Source: CAD feature listing. Evaluate the final solid. Frame: model axes, mm. Face numbers are marked on the shaded views. A direction names the side the tool comes from. Round coordinates to 2 decimals unless told otherwise and drop trailing zeros. Order: outer loops, then holes, each group sorted by start corner. A loop starts at its lowest first (then second) coordinate and runs counter-clockwise, first axis right, second up. Notation, with made-up numbers: M 27.5,63 L 44.5,63 A13 cw 44.5,70 Z; hole C 73.25,-23 d11. An arc over 180 degrees is marked long. Answer in a Markdown table with one row per item. Add a question column.
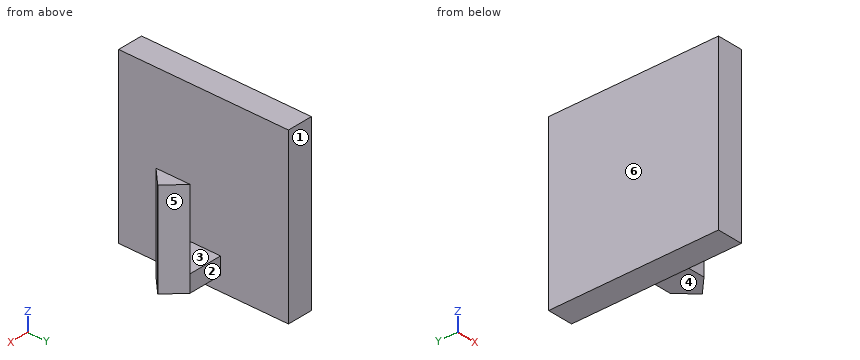
Autodesk Inventor part; units mm, degrees
ref_plane "YZ Plane" through (0, 0, 0) normal (1, 0, 0) x (0, 1, 0)
ref_plane "XZ Plane" through (0, 0, 0) normal (0, 1, 0) x (-1, 0, 0)
ref_plane "XY Plane" through (0, 0, 0) normal (0, 0, 1) x (1, 0, 0)
sketch "Esquisse1" plane through (0, 0, 0) normal (1, 0, 0) x (0, 1, 0)
  line L0 (5.4849, 2.6087) -> (-4.5151, 2.6087)
  line L1 (-4.5151, 2.6087) -> (-4.5151, -7.3913)
  line L2 (-4.5151, -7.3913) -> (5.4849, -7.3913)
  line L3 (5.4849, -7.3913) -> (5.4849, 2.6087)
  point P0 (0, 0)
  dimension "d0" = 10
  dimension "d1" = 10
extrude "Extrusion1" add sketch "Esquisse1" along normal blind 1.5
sketch "Esquisse2" plane through (1.5, 0, 0) normal (1, 0, 0) x (0, 0, -1)
  line L0 (5.5438, 1.4849) -> (6.5438, 1.4849)
  line L1 (6.5438, 1.4849) -> (6.5438, -0.5151)
  line L2 (6.5438, -0.5151) -> (5.5438, -0.5151)
  line L3 (5.5438, -0.5151) -> (5.5438, 1.4849)
  line L4 (7.3913, 5.4849) -> (-2.6087, 5.4849)
  point P0 (0, 0)
  dimension "d4" = 1
  dimension "d5" = 2
  dimension "d6" = 4
extrude "Extrusion2" add sketch "Esquisse2" along normal blind 2
sketch "Esquisse3" plane through (3.5, 0, 0) normal (1, 0, 0) x (0, 0, -1)
  line L0 (6.5438, 1.4849) -> (6.5438, -0.5151)
  line L1 (6.5438, 1.4849) -> (0.9284, 1.4849)
  line L2 (0.9284, 1.4849) -> (0.9284, -0.5151)
  line L3 (0.9284, -0.5151) -> (6.5438, -0.5151)
  line L4 (6.5438, -0.5151) -> (6.5438, 1.4849)
  point P0 (0, 0)
extrude "Extrusion3" add sketch "Esquisse3" along normal blind 1
chamfer "Chanfrein1" distance 1 angle 45 2 edges at (4.5, 1.4849, -3.7361) (4.5, -0.5151, -3.7361)
properties part number "crochet"
(1) Line query: line 1 (X direction, y = 4.5, z = 0.5); line 2 (Z direction, x = 2.85, y = 0.75); line 3 (Z direction, x = 3.65, y = 0.25). Output: solid intervals per line, ascending. Write a range as from..to.
(2) Cut plane C-C (x = 1.9). Return loops of the section in (y, z), and give its area (3 significant figures).
(3) Draft query along X for the marked faces 3, 4, 5 and 6. Return one class per face: +X half, -X half, draft (parallel to the pull), parting line (faces both ways), or undercut.
(4) Access query for the marked faces 1 and 2. Directions: +Z, -Z, +X, -X, +Y, -Y. A direction counts if a zero-diameter tool reaches every point of the face in a straight line with its end or side. Return the directions, or none.
(5) Pin query (flat end, axial travel): pin 1 (4 mm diameter, centred on y = -2, z = -4.5, fed in from +X); pin 2 (3 mm diameter, centred on y = 3.5, z = -5, fed in from +X); pin 3 (1.1 mm diameter, centred on x = 4, y = 0.5, fed in from +Z). Return the tip coordinate at first contact, or that it passes through.
(6) Cut plane D-D (y = 2.5). Return loops of the section in (x, z).
Answer list:
| question | item | result |
|---|---|---|
| 1 | line 1 | 0..1.5 |
| 1 | line 2 | -6.54..-5.54 |
| 1 | line 3 | -6.54..-0.93 |
| 2 | outline | M -0.52,-6.54 L 1.48,-6.54 L 1.48,-5.54 L -0.52,-5.54 Z |
| 2 | area | 2.00 mm² |
| 3 | face 3 | undercut |
| 3 | face 4 | draft |
| 3 | face 5 | +X half |
| 3 | face 6 | -X half |
| 4 | face 1 | +Z, -Z, +X, -X, +Y |
| 4 | face 2 | +Z, -Z, +X, +Y |
| 5 | pin 1 | x = 4.02 |
| 5 | pin 2 | x = 1.5 |
| 5 | pin 3 | z = -0.93 |
| 6 | outline | M 0,-7.39 L 1.5,-7.39 L 1.5,2.61 L 0,2.61 Z |
